```python
from build123d import *

# Parameters (mm, degrees)
ESQUISSE2_R             = 10.397646043
ESQUISSE2_R_2           = 5
BOSS_EXTRU_1_DEPTH      = 44
ESQUISSE3_R             = 9.441003055
BOSS_EXTRU_2_DEPTH      = 10
ESQUISSE4_R             = 2.5
ENL_V_MAT_EXTRU_1_DEPTH = 111


with BuildPart() as part:
    # Esquisse1 → Révolution1 (revolve)
    with BuildSketch(Plane.XY, mode=Mode.PRIVATE) as r_volution1_sk:
        with BuildLine():
            Line((-35, 50), (-30, 50))
            Line((-30, 50), (29.961005428, 50))
            ThreePointArc((29.961005428, 50), (20.217405473, 26.236864796), (0, 10.397646043))
            Line((0, 10.397646043), (0, 5))
            ThreePointArc((0, 5), (23.755589554, 22.634541458), (35, 50))
            Line((35, 50), (35, 50.592048887))
            Line((35, 50.592048887), (35, 64))
            Line((35, 64), (30, 64))
            Line((30, 64), (30, 63.944286902))
            ThreePointArc((30, 63.944286902), (27.966065457, 59.033934543), (23.055713098, 57))
            Line((23.055713098, 57), (9.532038357, 57))
            Line((9.532038357, 57), (-9.532038357, 57))
            Line((-9.532038357, 57), (-23.055713098, 57))
            ThreePointArc((-23.055713098, 57), (-27.966065457, 59.033934543), (-30, 63.944286902))
            Line((-30, 63.944286902), (-30, 64))
            Line((-30, 64), (-35, 64))
            Line((-35, 64), (-35, 50.592048887))
            Line((-35, 50.592048887), (-35, 50))
        make_face()
    revolve(r_volution1_sk.sketch.rotate(Axis((0, 0, 0), (1, 0, 0)), 90), axis=Axis((0, 0, 0), (1, 0, 0)))

    # Esquisse2 → Boss.-Extru.1 (add)
    with BuildSketch(Plane.ZY.offset(35)):
        Circle(ESQUISSE2_R)
        Circle(ESQUISSE2_R_2, mode=Mode.SUBTRACT)
    extrude(amount=-BOSS_EXTRU_1_DEPTH)

    # Esquisse3 → Boss.-Extru.2 (add)
    with BuildSketch(Plane(origin=(9, 0, 0), x_dir=(0, 0, -1), z_dir=(1, 0, 0))):
        Circle(ESQUISSE3_R)
    extrude(amount=-BOSS_EXTRU_2_DEPTH)

    # Esquisse4 → Enlèv. mat.-Extru.1 (cut)
    with BuildSketch(Plane(origin=(35, 0, 0), x_dir=(0, 0, -1), z_dir=(1, 0, 0))):
        with Locations(Location((0, 26.02006747, 0), (0, 0, 309.751623476))):
            Circle(ESQUISSE4_R)
        with Locations(Location((27.487866147, 0, 0), (0, 0, 289.434771235))):
            Circle(ESQUISSE4_R)
        with Locations(Location((-29.26701606, 0, 0), (0, 0, 359.999999748))):
            Circle(ESQUISSE4_R)
    extrude(amount=-ENL_V_MAT_EXTRU_1_DEPTH, mode=Mode.SUBTRACT)


solid = part.part
```
Could you check a few things on this model? Use its own coordinates, in mm. A direction names the side the tool comes from. Round coordinates to 2 decimals unless told otherwise and drop trailing zeros. Answer in a Markdown table with one row per item. Add a question column.
Q1. Will these pins go through, and if not, where does the flat tip stop? pin 1 Ø6 at (x, z) = (20, -25.5) entering from -Y; pin 2 Ø8 at (y, z) = (-1, 28.5) entering from +X; pin 3 Ø4 at (y, z) = (-30, 34.5) entering from -X.
Q2. If I drill on line 1 (Y direction, x = -23, z = 0); line 2 (Z direction, x = 7.5, y = 11) (3 decimals); line 3 (Y direction, x = 25.5, z = 0), over which ranges is the centre line in solid material (lowest first)? Write a range as from..to.
Q3. On a 3-axis mill with a long thin cutter (end or side, diameter ignored), from which of +Z, -Z, +X, -X, +Y, -Y can I reach the whole of each face in a straight line? I mean faces 1 (the cylindrical face through (32.47, 62.48, -13.87)), 2 (the flat face through (9, 0, 0)), 3 (the flat face through (-1, 0, 0)). Say none if no direction works.
Q4. Imagine slicing it at A-A (y = 0). Give the number of separate pieces and of enclosed holes in the cut face, then the cut area to 3 significant figures.
Q5. If we mould it in two halves opening along Z, with no side actions, what happens to faces 4 (the flat face through (-35, -2, -5)), 5 (the cylindrical face through (25.1, 0.8, 26.9)), 6 (the cylindrical face through (-0.32, 50.57, 26.3))? For each: +Z half, -Z half, draft (parallel to the pull), parting line (faces both ways), or undercut.
Values:
| question | item | result |
|---|---|---|
| 1 | pin 1 | y = -52.37 |
| 1 | pin 2 | x = 29.89 |
| 1 | pin 3 | x = 28.72 |
| 2 | line 1 | -57..-50, -10.4..-5, 5..10.4, 50..57 |
| 2 | line 2 | -55.929..-48.775, -9.301..9.301, 48.775..55.929 |
| 2 | line 3 | -57.44..-50, -34.93..-25.01, 28.52..34.93, 50..57.44 |
| 3 | face 1 | +X, -X |
| 3 | face 2 | +X |
| 3 | face 3 | -X |
| 4 | separate pieces | 3 |
| 4 | enclosed holes | 0 |
| 4 | area | 2,180 mm^2 |
| 5 | face 4 | draft |
| 5 | face 5 | undercut |
| 5 | face 6 | parting line |
